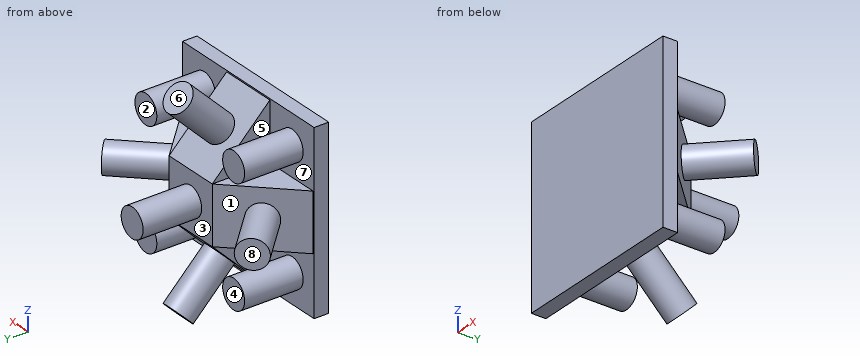
from build123d import *

# Parameters (mm, degrees)
SKETCH1_W           = 152.4
SKETCH1_H           = 152.4
BOSS_EXTRUDE1_DEPTH = 12.7
SKETCH2_R           = 12.7
BOSS_EXTRUDE2_DEPTH = 50.8
BOSS_EXTRUDE3_DEPTH = 50
CUT_EXTRUDE1_DEPTH  = 50
CUT_EXTRUDE2_DEPTH  = 50
SKETCH6_R           = 12.7
BOSS_EXTRUDE4_DEPTH = 50.8
SKETCH7_R           = 12.7
BOSS_EXTRUDE5_DEPTH = 50.8
SKETCH8_R           = 12.7
BOSS_EXTRUDE6_DEPTH = 50.8
SKETCH9_R           = 12.7
BOSS_EXTRUDE7_DEPTH = 50.8
SKETCH10_R          = 12.7
BOSS_EXTRUDE8_DEPTH = 50.8


with BuildPart() as part:
    # Sketch1 → Boss-Extrude1 (new body)
    with BuildSketch(Plane(origin=(0, 0, 0), x_dir=(1, 0, 0), z_dir=(0, 1, 0))):
        with Locations((76.2, 76.2)):
            Rectangle(SKETCH1_W, SKETCH1_H)
    extrude(amount=-BOSS_EXTRUDE1_DEPTH)

    # Sketch2 → Boss-Extrude2 (add)
    with BuildSketch(Plane(origin=(0, 0, 0), x_dir=(1, 0, 0), z_dir=(0, 1, 0))):
        with Locations(Location((25.4, 127, 0), (0, 0, 270))):
            Circle(SKETCH2_R)
        with Locations(Location((127, 127, 0), (0, 0, 270))):
            Circle(SKETCH2_R)
        with Locations(Location((127, 25.4, 0), (0, 0, 270))):
            Circle(SKETCH2_R)
        with Locations(Location((25.4, 25.4, 0), (0, 0, 270))):
            Circle(SKETCH2_R)
    extrude(amount=BOSS_EXTRUDE2_DEPTH)

    # Sketch3 → Boss-Extrude3 (add)
    with BuildSketch(Plane(origin=(0, 0, 0), x_dir=(1, 0, 0), z_dir=(0, 1, 0))):
        Polygon((51.2, 151.2), (51.2, 101.2), (1.2, 101.2), (1.2, 51.2), (51.2, 51.2), (51.2, 1.2), (101.2, 1.2), (101.2, 51.2), (151.2, 51.2), (151.2, 101.2), (101.2, 101.2), (101.2, 151.2), align=None)
    extrude(amount=BOSS_EXTRUDE3_DEPTH)

    # Sketch4 → Cut-Extrude1 (cut)
    with BuildSketch(Plane.XY.offset(-51.2)):
        Polygon((1.2, 0), (51.2, 50), (1.2, 50), align=None)
        Polygon((101.2, 50), (151.2, 0), (151.2, 50), align=None)
    extrude(amount=-CUT_EXTRUDE1_DEPTH, mode=Mode.SUBTRACT)

    # Sketch5 → Cut-Extrude2 (cut)
    with BuildSketch(Plane(origin=(101.2, 0, 0), x_dir=(0, 0, -1), z_dir=(1, 0, 0))):
        Polygon((1.2, 0), (51.2, 50), (1.2, 50), align=None)
        Polygon((101.2, 50), (151.2, 0), (151.2, 50), align=None)
    extrude(amount=-CUT_EXTRUDE2_DEPTH, mode=Mode.SUBTRACT)

    # Sketch6 → Boss-Extrude4 (add)
    with BuildSketch(Plane(origin=(75.6, 75.6, 0), x_dir=(0, 0, -1), z_dir=(0.7071067811865475, 0.7071067811865477, 0))):
        with Locations(Location((76.2, -71.559206256, 0), (0, 0, 270))):
            Circle(SKETCH6_R)
    extrude(amount=BOSS_EXTRUDE4_DEPTH)

    # Sketch7 → Boss-Extrude5 (add)
    with BuildSketch(Plane(origin=(0, 75.6, -75.6), x_dir=(1, 0, 0), z_dir=(0, 0.7071067811865476, -0.7071067811865475))):
        with Locations(Location((76.2, 71.559206256, 0), (0, 0, 90))):
            Circle(SKETCH7_R)
    extrude(amount=BOSS_EXTRUDE5_DEPTH)

    # Sketch8 → Boss-Extrude6 (add)
    with BuildSketch(Plane(origin=(0.6, -0.6, 0), x_dir=(0, 0, 1), z_dir=(-0.7071067811865476, 0.7071067811865475, 0))):
        with Locations(Location((-76.2, 36.203867197, 0), (0, 0, 90))):
            Circle(SKETCH8_R)
    extrude(amount=BOSS_EXTRUDE6_DEPTH)

    # Sketch9 → Boss-Extrude7 (add)
    with BuildSketch(Plane(origin=(0, -0.6, -0.6), x_dir=(1, 0, 0), z_dir=(0, 0.7071067811865477, 0.7071067811865475))):
        with Locations(Location((76.2, 36.203867197, 0), (0, 0, 90))):
            Circle(SKETCH9_R)
    extrude(amount=BOSS_EXTRUDE7_DEPTH)

    # Sketch10 → Boss-Extrude8 (add)
    with BuildSketch(Plane(origin=(0, 50, 0), x_dir=(1, 0, 0), z_dir=(0, 1, 0))):
        with Locations(Location((76.2, 76.2, 0), (0, 0, 270))):
            Circle(SKETCH10_R)
    extrude(amount=BOSS_EXTRUDE8_DEPTH)


solid = part.part
Geometry check sheet. Reference: the model listing, model coordinates, mm. Face numbers are marked on the shaded views. A direction names the side the tool comes from. Coordinates: 2 decimals unless noted, no trailing zeros. Order: outer loops, then holes, each group sorted by start corner. A loop starts at its lowest first (then second) coordinate and runs counter-clockwise, first axis right, second up. Notation, with made-up numbers: (67, -8) - (119, -8) arc R20 ccw to (119, 27) - close; hole circle Ø5 at (1.5, 40.5). An arc over 180 degrees is marked (long way). Answer in a Markdown table with one row per item. Add a question column.
1) Cross-section at A-A, the plane x = 94.5. Record the cut outline in (y, z).
2) Cross-section at B-B, the plane z = -69. Record the cut outline in (x, y).
3) Set-up check for the marked faces 1, 2, 3, 4 and 5: record each of +Z, -Z, +X, -X, +Y, -Y from which the full face is reachable in a straight line by a thin tool's end or side.
4) Cross-section at D-D, the plane z = -98. Record the cut outline in (x, y), then the cut area to 3 significant figures.
5) Release check for a two-part mould opening along Z. For the marked faces 6, 7 and 8 record: +Z half, -Z half, draft (parallel to the pull), parting line (faces both ways), or undercut.
6) Material ranges on line 1 along X through (y, z) = (33, -117.5); line 2 along Z through (x, y) = (20, 39); line 3 along X through (y, z) = (40.5, -44), recorded low to high. Write a range as [from, to].
7) Cross-section at C-C, the plane y = 60. State how many separate pieces and enclosed holes the cut face has, then the cut area to 3 significant figures.
8) Gauge pin test, flat ends, axial feed: P1, Ø8, axis at x = 70.5, y = 19, coming from the -Z side; P2, Ø25, axis at y = 29, z = -16, coming from the -X side; P3, Ø7.5, axis at x = 22, z = -130, coming from the +Y side; P4, Ø1.5, axis at x = 89.5, z = -75, coming from the +Y side. Record the tip position at first contact, or that the pin passes through.
Check result:
| question | item | result |
|---|---|---|
| 1 | outline | (-12.7, -152.4) - (0, -152.4) - (0, -151.2) - (50, -101.2) - (50, -51.2) - (0, -1.2) - (0, 0) - (-12.7, 0) - close |
| 2 | outline | (-17.12, 53.52) - (18.8, 17.6) - (1.2, 0) - (0, 0) - (0, -12.7) - (152.4, -12.7) - (152.4, 0) - (151.2, 0) - (133.6, 17.6) - (169.52, 53.52) - (154.72, 68.32) - (118.8, 32.4) - (101.2, 50) - (86.66, 50) - (86.66, 100.8) - (65.74, 100.8) - (65.74, 50) - (51.2, 50) - (33.6, 32.4) - (-2.32, 68.32) - close |
| 3 | face 1 | none |
| 3 | face 2 | +Z, +X, +Y |
| 3 | face 3 | +Y |
| 3 | face 4 | -Z, -X, +Y |
| 3 | face 5 | +Z, +Y |
| 4 | outline | (0, -12.7) - (152.4, -12.7) - (152.4, 0) - (151.2, 0) - (101.2, 50) - (51.2, 50) - (1.2, 0) - (0, 0) - close |
| 4 | area | 6,940 mm² |
| 5 | face 6 | +Z half |
| 5 | face 7 | undercut |
| 5 | face 8 | draft |
| 6 | line 1 | x = [16.97, 33.83], [51.2, 101.2], [118.57, 135.43] |
| 6 | line 2 | z = [-138.49, -115.51], [-87.64, -64.76], [-36.89, -13.91] |
| 6 | line 3 | x = [51.2, 101.2] |
| 7 | separate pieces | 5 |
| 7 | enclosed holes | 0 |
| 7 | area | 2,130 mm² |
| 8 | P1 | stops at z = -140.87 |
| 8 | P2 | stops at x = 12.7 |
| 8 | P3 | stops at y = 50.8 |
| 8 | P4 | stops at y = 100.8 |
